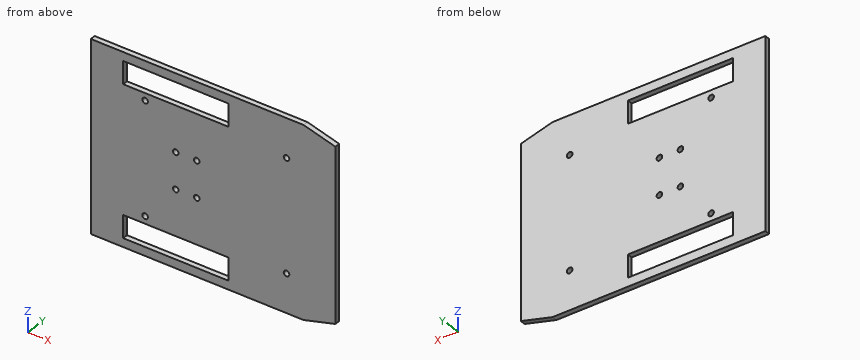
```python
from build123d import *

# Parameters (mm, degrees)
SKETCH1_W           = 110
SKETCH1_H           = 90
BOSS_EXTRUDE1_DEPTH = 3
SKETCH2_W           = 60
SKETCH2_H           = 8.5
SKETCH2_R           = 1.6
CUT_EXTRUDE1_DEPTH  = 3
SKETCH4_R           = 1.6
CUT_EXTRUDE2_DEPTH  = 10
BOSS_EXTRU_1_DEPTH  = 3


with BuildPart() as part:
    # Sketch1 → Boss-Extrude1 (new body)
    with BuildSketch(Plane(origin=(0, 0, 0), x_dir=(1, 0, 0), z_dir=(0, 1, 0))):
        with Locations((55, 45)):
            Rectangle(SKETCH1_W, SKETCH1_H)
    extrude(amount=BOSS_EXTRUDE1_DEPTH)

    # Sketch2 → Cut-Extrude1 (cut)
    with BuildSketch(Plane(origin=(0, 3, 0), x_dir=(1, 0, 0), z_dir=(0, 1, 0))):
        with Locations((40, 85.75)):
            Rectangle(SKETCH2_W, SKETCH2_H)
        with Locations((40, 4.25)):
            Rectangle(SKETCH2_W, SKETCH2_H)
        with Locations(Location((40, 55.4, 0), (0, 0, 270))):
            Circle(SKETCH2_R)
        with Locations(Location((52, 55.4, 0), (0, 0, 270))):
            Circle(SKETCH2_R)
        with Locations(Location((52, 34.6, 0), (0, 0, 270))):
            Circle(SKETCH2_R)
        with Locations(Location((40, 34.6, 0), (0, 0, 270))):
            Circle(SKETCH2_R)
    extrude(amount=-CUT_EXTRUDE1_DEPTH, mode=Mode.SUBTRACT)

    # Sketch4 → Cut-Extrude2 (cut)
    with BuildSketch(Plane(origin=(0, 3, 0), x_dir=(1, 0, 0), z_dir=(0, 1, 0))):
        with Locations(Location((22.5, 77.26, 0), (0, 0, 270))):
            Circle(SKETCH4_R)
        with Locations(Location((22.5, 12.74, 0), (0, 0, 270))):
            Circle(SKETCH4_R)
        with Locations(Location((103.27, 12.74, 0), (0, 0, 270))):
            Circle(SKETCH4_R)
        with Locations(Location((103.27, 77.26, 0), (0, 0, 270))):
            Circle(SKETCH4_R)
    extrude(amount=-CUT_EXTRUDE2_DEPTH, mode=Mode.SUBTRACT)

    # Esquisse1 → Boss.-Extru.1 (add)
    with BuildSketch(Plane(origin=(0, 3, 0), x_dir=(1, 0, 0), z_dir=(0, 1, 0))):
        Polygon((113, -9.466090987), (-8.5, -9.466090987), (-8.5, -4.466090987), (-8.5, 94.466090987), (-8.5, 99.466090987), (113, 99.466090987), (131.165303172, 94.5), (131.165303172, -4.5), align=None)
        Polygon((10, 0), (10, -4.466090987), (70, -4.466090987), (70, 0), (110, 0), (110, 90), (70, 90), (70, 94.466090987), (10, 94.466090987), (10, 90), (0, 90), (0, 0), align=None, mode=Mode.SUBTRACT)
    extrude(amount=-BOSS_EXTRU_1_DEPTH)


solid = part.part
```
Model file for the job. Use its own axes, mm. Coordinates: 2 decimals unless noted, no trailing zeros. Write each loop counter-clockwise with the first axis right and the second up, starting at its lowest first coordinate (ties: lowest second). Pieces come first, ordered by that corner, then holes. Notation, with made-up numbers: (40, 2.25) - (95, 2.25) arc R21 ccw to (95, 34.25) - close; hole circle Ø3 at (88, 29). An arc over 180 degrees is marked (long way). One line per question, with ' | ' between items. Start each with the question number.
Q1. Drill centre lines: line 1 (Z direction, x = 103.27, y = 1.5); line 2 (X direction, y = 2, z = -34.6); line 3 (Z direction, x = 12, y = 2.1). Where is each one in solid material? Low to high. Write a range as [from, to].
Q2. Cut at D-D, the plane y = 2.25. Give the number of separate pieces and of enclosed holes in the cut face, then the cut area to 3 significant figures.
Q3. Cut at B-B, the plane z = -12.74. List the corners of the cut face in (x, y), then the cut area to 3 significant figures.
Q4. Cut at A-A, the plane x = 22.5. List the corners of the cut face in (y, z).
Q5. Cut at C-C, the plane x = 103.27. List the corners of the cut face in (y, z).
Answer below:
1) line 1: [-99.47, -78.86], [-75.66, -14.34], [-11.14, 9.47] | line 2: [-8.5, 38.4], [41.6, 50.4], [53.6, 131.17] | line 3: [-99.47, -94.47], [-81.5, -8.5], [4.47, 9.47]
2) separate pieces: 1 | enclosed holes: 10 | area: 13,500 mm^2
3) outline: (-8.5, 0) - (20.9, 0) - (20.9, 3) - (-8.5, 3) - close; (24.1, 0) - (101.67, 0) - (101.67, 3) - (24.1, 3) - close; (104.87, 0) - (131.17, 0) - (131.17, 3) - (104.87, 3) - close | area: 400 mm^2
4) outline: (0, -99.47) - (3, -99.47) - (3, -94.47) - (0, -94.47) - close; (0, -81.5) - (3, -81.5) - (3, -78.86) - (0, -78.86) - close; (0, -75.66) - (3, -75.66) - (3, -14.34) - (0, -14.34) - close; (0, -11.14) - (3, -11.14) - (3, -8.5) - (0, -8.5) - close; (0, 4.47) - (3, 4.47) - (3, 9.47) - (0, 9.47) - close
5) outline: (0, -99.47) - (3, -99.47) - (3, -78.86) - (0, -78.86) - close; (0, -75.66) - (3, -75.66) - (3, -14.34) - (0, -14.34) - close; (0, -11.14) - (3, -11.14) - (3, 9.47) - (0, 9.47) - close
